Design review of the part built by this model. Coordinates are the model's own, in mm. Face numbers are marked on the shaded views. A direction names the side the tool comes from. Coordinates: 2 decimals unless noted, no trailing zeros. Loops run counter-clockwise (first coordinate to the right, second up) from the corner with the lowest first, then second, coordinate; pieces in that order, holes last. Notation, with made-up numbers: (72.25, 52) -> (117.25, 52) arc R15 cw to (117.25, 63) -> close; hole circle Ø4 at (-30.75, 53). An arc over 180 degrees is marked (long way). Use a Markdown table: item, result. Add a question column.
Q1. Take a section at A-A on z = -3.75. Write out the cut boundary in (x, y).
Q2. For the marked faces 1, 2, 3 and 4, list the 3-axis set-ups (+Z, -Z, +X, -X, +Y, -Y) from which the entire face can be reached by the end or side of a thin tool; tool diameter is ignored.
Q3. Take a section at D-D on y = -135.5. Write out the cut boundary in (x, z), plus the area to 3 significant figures.
Q4. Clearance check with flat-ended pins moving along their axes: pin 1 Ø1.8 at (x, y) = (18.5, -150) entering from +Z; pin 2 Ø3 at (x, y) = (19.5, -131) entering from +Z; pin 3 Ø10 at (x, y) = (0, -125) entering from -Z. State where each tip first meets the part, or that it passes through.
Q5. For probe 1 along Y at (x, z) = (0, 7.25); probe 2 along X at (y, z) = (-145, 3.05); probe 3 along Z at (x, y) = (1, -130), list the stretches that pass through material, from the lowest coordinate up.
Q6. Take a section at C-C on x = 32. Write out the cut boundary in (y, z), plus the area to 3 significant figures.
Q7. Take a section at B-B on y = -125. Write out the cut boundary in (x, z).
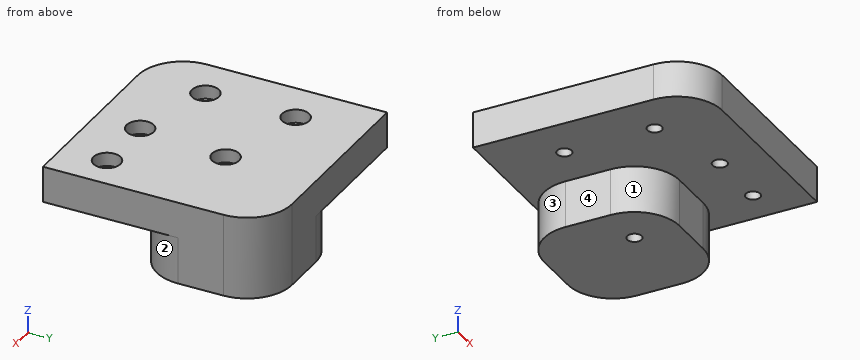
from build123d import *

# Parameters (mm, degrees)
SKETCH_1_R          = 1.6
EXTRUDE_1_DEPTH     = 8
SKETCH_2_R          = 3
CUT_EXTRUDE_1_DEPTH = 3
FILLET_1_R          = 10
SKETCH_3_R          = 1.6
EXTRUDE_2_DEPTH     = 18.3999492
SKETCH_4_R          = 3
CUT_EXTRUDE_2_DEPTH = 3
FILLET_2_R          = 10


with BuildPart() as part:
    # 草图1 → 凸台-拉伸1 (new body)
    with BuildSketch(Plane.XY):
        Polygon((-10, -110), (10, -110), (10, -140.028839027), (40, -140.028839027), (40, -160), (-10, -160), align=None)
        with Locations((0, -125)):
            Circle(SKETCH_1_R, mode=Mode.SUBTRACT)
        with Locations((0, -145)):
            Circle(SKETCH_1_R, mode=Mode.SUBTRACT)
        with Locations((18, -150.014419513)):
            Circle(SKETCH_1_R, mode=Mode.SUBTRACT)
        with Locations((32, -150.014419513)):
            Circle(SKETCH_1_R, mode=Mode.SUBTRACT)
    extrude(amount=EXTRUDE_1_DEPTH)

    # 草图2 → 切除-拉伸1 (cut)
    with BuildSketch(Plane.XY.offset(8)):
        with Locations((32, -150.014419513)):
            Circle(SKETCH_2_R)
        with Locations((18, -150.014419513)):
            Circle(SKETCH_2_R)
        with Locations((0, -145)):
            Circle(SKETCH_2_R)
        with Locations((0, -125)):
            Circle(SKETCH_2_R)
    extrude(amount=-CUT_EXTRUDE_1_DEPTH, mode=Mode.SUBTRACT)

    # 圆角1
    fillet_1_edges = [part.edges().sort_by_distance(p)[0] for p in [
        (10, -140.028839027, 4),
        (-10, -160, 4),
    ]]
    fillet(fillet_1_edges, radius=FILLET_1_R)

    # 草图3 → 凸台-拉伸2 (add)
    with BuildSketch(Plane.XY.offset(8)):
        with BuildLine():
            Line((10, -130.028839027), (10, -110))
            Line((10, -110), (40, -110))
            Line((40, -110), (40, -140.028839027))
            Line((40, -140.028839027), (20, -140.028839027))
            ThreePointArc((20, -140.028839027), (12.928932188, -137.099906839), (10, -130.028839027))
        make_face()
        with Locations((20, -130.028839027)):
            Circle(SKETCH_3_R, mode=Mode.SUBTRACT)
    extrude(amount=-EXTRUDE_2_DEPTH)

    # 草图4 → 切除-拉伸2 (cut)
    with BuildSketch(Plane.XY.offset(8)):
        with Locations((20, -130.028839027)):
            Circle(SKETCH_4_R)
    extrude(amount=-CUT_EXTRUDE_2_DEPTH, mode=Mode.SUBTRACT)

    # 圆角2
    fillet_2_edges = [part.edges().sort_by_distance(p)[0] for p in [
        (40, -140.028839027, -5.1999746),
        (40, -110, -1.1999746),
        (10, -110, -5.1999746),
    ]]
    fillet(fillet_2_edges, radius=FILLET_2_R)


solid = part.part
Answer list:
| question | item | result |
|---|---|---|
| 1 | outline | (10, -130.03) arc R10 ccw to (20, -140.03) -> (30, -140.03) arc R10 ccw to (40, -130.03) -> (40, -120) arc R10 ccw to (30, -110) -> (20, -110) arc R10 ccw to (10, -120) -> close; hole circle Ø3.2 at (20, -130.03) |
| 2 | face 1 | -Z, -X, -Y |
| 2 | face 2 | -Z, +X, -Y |
| 2 | face 3 | -Z, -X, +Y |
| 2 | face 4 | -Z, -X, +Y, -Y |
| 3 | outline | (-10, 0) -> (11.63, 0) -> (11.63, -10.4) -> (38.37, -10.4) -> (38.37, 0) -> (40, 0) -> (40, 8) -> (-10, 8) -> close |
| 3 | area | 678 mm² |
| 4 | pin 1 | through |
| 4 | pin 2 | z = 5 |
| 4 | pin 3 | z = 0 |
| 5 | probe 1 | -160 to -148, -142 to -128, -122 to -110 |
| 5 | probe 2 | -10 to -1.6, 1.6 to 40 |
| 5 | probe 3 | 0 to 8 |
| 6 | outline | (-160, 0) -> (-151.61, 0) -> (-151.61, 5) -> (-153.01, 5) -> (-153.01, 8) -> (-160, 8) -> close; (-148.41, 0) -> (-139.83, 0) -> (-139.83, -10.4) -> (-110.2, -10.4) -> (-110.2, 8) -> (-147.01, 8) -> (-147.01, 5) -> (-148.41, 5) -> close |
| 6 | area | 672 mm² |
| 7 | outline | (-10, 0) -> (-1.6, 0) -> (-1.6, 5) -> (-3, 5) -> (-3, 8) -> (-10, 8) -> close; (1.6, 0) -> (10, 0) -> (10, -10.4) -> (40, -10.4) -> (40, 8) -> (3, 8) -> (3, 5) -> (1.6, 5) -> close |
